Geometry check sheet. Reference: the model listing, model coordinates, mm. A direction names the side the tool comes from. Coordinates: 2 decimals unless noted, no trailing zeros. Write each loop counter-clockwise with the first axis right and the second up, starting at its lowest first coordinate (ties: lowest second). Pieces come first, ordered by that corner, then holes. Notation, with made-up numbers: (80, 65) -> (116, 65) arc R30 cw to (116, 87) -> close; hole circle Ø8 at (36, 39). An arc over 180 degrees is marked (long way). Put each result on its own line as item: value. Start each with the question number.
from build123d import *

# Parameters (mm, degrees)
F2_R     = 31.75
F2_R_2   = 21.59
F3_DEPTH = 44.45
F2_R_3   = 50.8
F4_DEPTH = 101.6


# Not quite as in the source:
# - a variable given as a bare number and used for a length is read in inches; the dataset says mm whatever the document's units were


with BuildPart() as f3:
    # F2 (on Front) → F3 (new body, symmetric)
    with BuildSketch(Plane.XZ):
        Circle(F2_R)
        Circle(F2_R_2, mode=Mode.SUBTRACT)
    extrude(amount=F3_DEPTH, both=True)

    # F2 (on Front) → F4 (join, symmetric)
    with BuildSketch(Plane.XZ):
        Circle(F2_R_3)
        Circle(F2_R, mode=Mode.SUBTRACT)
    extrude(amount=F4_DEPTH, both=True)


solid = f3.part
Item 1: Section check B-B, the plane z = 0. Enter the section's corners in (x, y), and give its area (3 significant figures).
Item 2: Access from +Z, -Z, +X, -X, +Y, -Y to the whole of each face (thin tool, end or side, straight path). Record for faces 1 (the cylindrical face through (-6.883, -72.625, -30.995)), 2 (the flat face through (21, 44.45, -7)), 3 (the flat face through (21.9, -101.6, 23.3)).
Item 3: Section check A-A, the plane x = 0. Enter the section's corners in (y, z), and give its area (3 significant figures).
Item 4: Go/stop test with flat-tipped pins: P1, Ø3, axis at x = 18.5, y = -75, coming from the +Z side; P2, Ø1.5, axis at x = 7, y = -48.5, coming from the -Z side; P3, Ø19, axis at x = -15, z = -14, coming from the -Y side. Record where each tip stops, or that it passes through.
Item 5: Scan lines: line 1 along Z through (x, y) = (0, -77); line 2 along Z through (x, y) = (0, 16); line 3 along X through (y, z) = (60.5, -5). Record each from-to range of solid material in increasing order. Write a range as [from, to].
Item 6: Section check D-D, the plane z = -43. Enter the section's corners in (x, y), and give its area (3 significant figures).
Item 7: Section check C-C, the plane y = -1.5. Enter the section's corners in (x, z).
Item 8: Mould release check, pull along Z, two halves, no side actions. Record for faces 4 (the flat face through (21, -44.45, -7)), 5 (the cylindrical face through (-11.012, -1.422, -49.592)), 6 (the cylindrical face through (-6.883, 73.425, -30.995)), 7 (the flat face through (21.9, 101.6, 23.3)): released by +Z, released by -Z, zero draft, split by the parting line, or undercut.
From the geometry:
1. outline: (-50.8, -101.6) -> (-31.75, -101.6) -> (-31.75, -44.45) -> (-21.59, -44.45) -> (-21.59, 44.45) -> (-31.75, 44.45) -> (-31.75, 101.6) -> (-50.8, 101.6) -> close; (21.59, -44.45) -> (31.75, -44.45) -> (31.75, -101.6) -> (50.8, -101.6) -> (50.8, 101.6) -> (31.75, 101.6) -> (31.75, 44.45) -> (21.59, 44.45) -> close
1. area: 9,550 mm²
2. face 1: -Y
2. face 2: +Y
2. face 3: +Z, -Z, +X, -X, -Y
3. outline: (-101.6, -50.8) -> (101.6, -50.8) -> (101.6, -31.75) -> (44.45, -31.75) -> (44.45, -21.59) -> (-44.45, -21.59) -> (-44.45, -31.75) -> (-101.6, -31.75) -> close; (-101.6, 31.75) -> (-44.45, 31.75) -> (-44.45, 21.59) -> (44.45, 21.59) -> (44.45, 31.75) -> (101.6, 31.75) -> (101.6, 50.8) -> (-101.6, 50.8) -> close
3. area: 9,550 mm²
4. P1: z = 47.87
4. P2: z = -50.41
4. P3: y = -44.45
5. line 1: [-50.8, -31.75], [31.75, 50.8]
5. line 2: [-50.8, -21.59], [21.59, 50.8]
5. line 3: [-50.55, -31.35], [31.35, 50.55]
6. outline: (-27.05, -101.6) -> (27.05, -101.6) -> (27.05, 101.6) -> (-27.05, 101.6) -> close
6. area: 11,000 mm²
7. outline: circle Ø101.6 at (0, 0); hole circle Ø43.18 at (0, 0)
8. face 4: undercut
8. face 5: split by the parting line
8. face 6: undercut
8. face 7: zero draft
